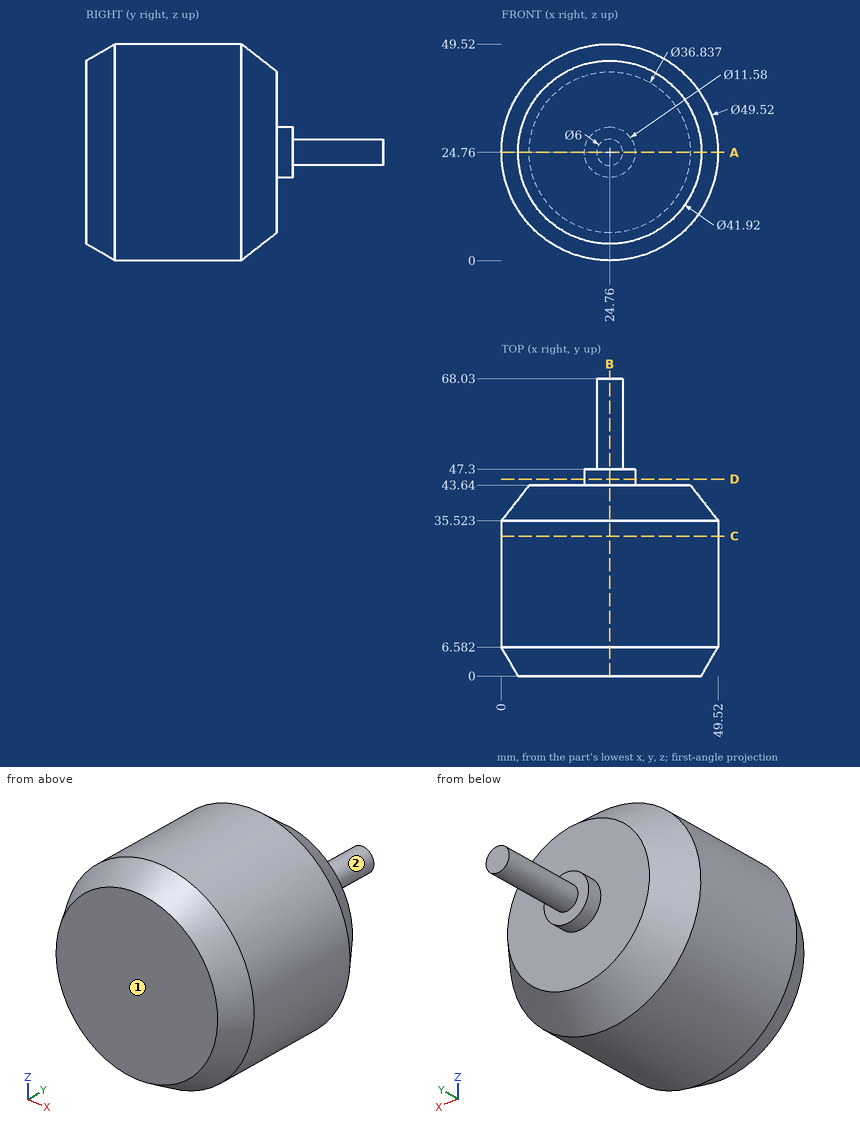
Design review of the part shown in the three views and the two pictorial views. Dimensions are in mm from the part's minimum x, y and z. A direction names the side the tool comes from. Coordinates: 2 decimals unless noted, no trailing zeros. Order: outer loops, then holes, each group sorted by start corner. A loop starts at its lowest first (then second) coordinate and runs counter-clockwise, first axis right, second up.
1) Clearance check with flat-ended pins moving along their axes: pin 1 (3 mm diameter, centred on x = 10, z = 24, fed in from +Y); pin 2 (10 mm diameter, centred on x = 29, y = 24.5, fed in from +Z); pin 3 (1.5 mm diameter, centred on y = 28, z = 25.5, fed in from -X); pin 4 (8 mm diameter, centred on y = 26.5, z = 32, fed in from +X). State where each tip first meets the part, or that it passes through.
2) Take a section at A-A, the plane z = 24.76. Give the boundary of the cut face in (x, y).
3) For the marked faces 1 and 2, list the 3-axis set-ups (+Z, -Z, +X, -X, +Y, -Y) from which the entire face can be reached by the end or side of a thin tool; tool diameter is ignored.
4) Wall thickness on line 1 along Y through (x, z) = (10.5, 13.5); line 2 along X through (y, z) = (22, 24); line 3 along Z through (x, y) = (24.5, 28): over which ranges is each line inside the solid? List them lowest first.
5) Take a section at B-B, the plane x = 24.76. Give the boundary of the cut face in (y, z).
6) Take a section at D-D, the plane y = 45. Give the boundary of the cut face in (x, z).
7) Take a section at C-C, the plane y = 32. Give the boundary of the cut face in (x, z).
Returned:
1. pin 1: stops at y = 43.64
1. pin 2: stops at z = 49.52
1. pin 3: stops at x = 0
1. pin 4: stops at x = 49.31
2. outline: (0, 6.58) - (3.8, 0) - (45.72, 0) - (49.52, 6.58) - (49.52, 35.52) - (43.18, 43.64) - (30.55, 43.64) - (30.55, 47.3) - (27.76, 47.3) - (27.76, 68.03) - (21.76, 68.03) - (21.76, 47.3) - (18.97, 47.3) - (18.97, 43.64) - (6.34, 43.64) - (0, 35.52) - close
3. face 1: +Z, -Z, +X, -X, -Y
3. face 2: +Y
4. line 1: y = 0 to 43.64
4. line 2: x = 0.01 to 49.51
4. line 3: z = 0 to 49.52
5. outline: (0, 3.8) - (6.58, 0) - (35.52, 0) - (43.64, 6.34) - (43.64, 18.97) - (47.3, 18.97) - (47.3, 21.76) - (68.03, 21.76) - (68.03, 27.76) - (47.3, 27.76) - (47.3, 30.55) - (43.64, 30.55) - (43.64, 43.18) - (35.52, 49.52) - (6.58, 49.52) - (0, 45.72) - close
6. outline: circle Ø11.58 at (24.76, 24.76)
7. outline: circle Ø49.52 at (24.76, 24.76)
